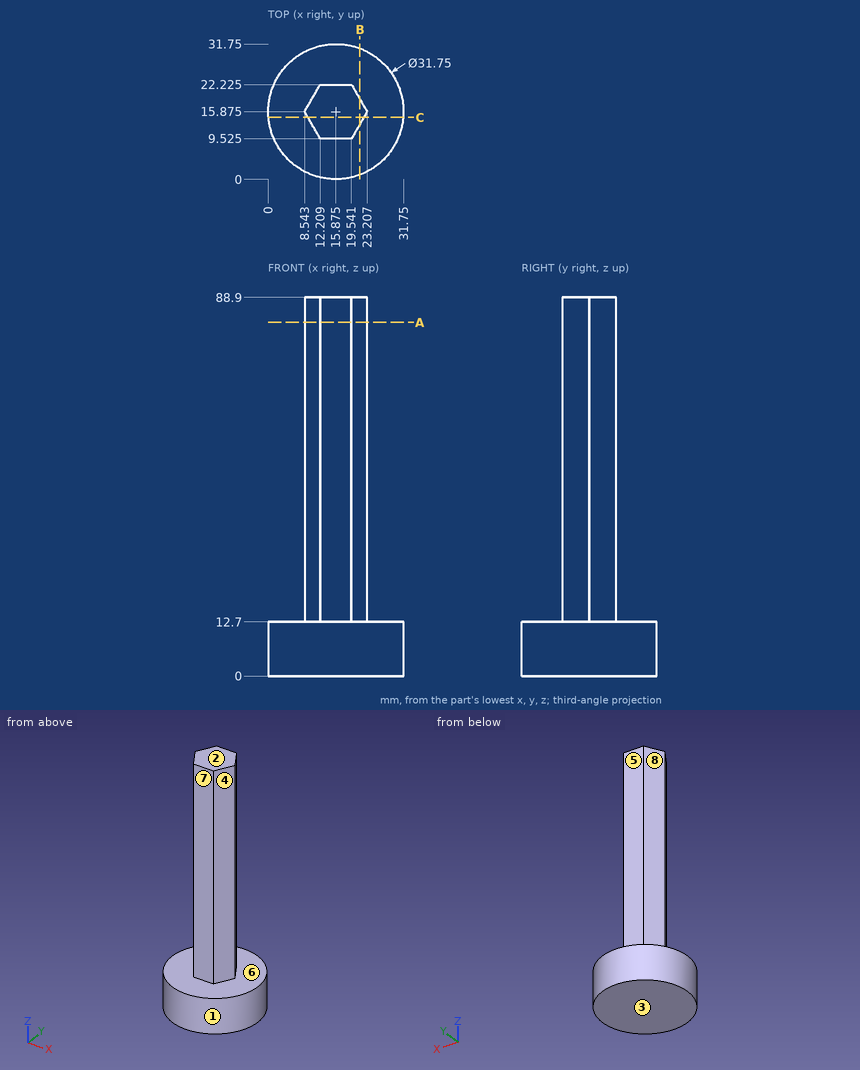
Geometry check sheet. Reference: drawing and pictorial views, mm from the part's lowest x, y, z. A direction names the side the tool comes from. Coordinates: 2 decimals unless noted, no trailing zeros. Order: outer loops, then holes, each group sorted by start corner. A loop starts at its lowest first (then second) coordinate and runs counter-clockwise, first axis right, second up. Notation, with made-up numbers: (77.5, -0.5) -> (101.5, -0.5) arc R21 cw to (101.5, 11.5) -> close; hole circle Ø2 at (77, 66.5). An arc over 180 degrees is marked (long way). Use CSV: the item, a comma, the result in double quotes. Start each with the question number.
Q1. Section check A-A, the plane z = 83. Record the cut outline in (x, y) (1 decimal), and give its area (3 significant figures).
Q2. Thickness scan on line 1 along Z through (x, y) = (27, 15); line 2 along Y through (x, z) = (13, 61.5) (1 decimal); line 3 along X through (y, z) = (17.5, 31.5). Record the ranges inside material, lowest first.
Q3. Tool access check on the marked faces 4, 5, 6, 7 and 8. Record the directions out of +Z, -Z, +X, -X, +Y, -Y that give a thin tool (end or side, any length) a straight path to the whole face; none if there is none.
Q4. Draft check along Z on the marked faces 1, 2 and 3. Enter one of: +Z half, -Z half, draft (parallel to the pull), parting line (faces both ways), or undercut.
Q5. Section check C-C, the plane y = 14.5. Record the cut outline in (x, z).
Q6. Depth check by flat-ended pin: P1, Ø8, axis at x = 6, y = 5.5, coming from the +Z side; P2, Ø1.5, axis at x = 25.5, z = 15, coming from the -Y side; P3, Ø4, axis at x = 21, z = 37, coming from the -Y side (3 decimals); P4, Ø3, axis at x = 7.5, z = 47, coming from the -Y side. Enter the tip coordinate at first touch or a pass-through.
Q7. Section check B-B, the plane x = 21.5. Record the cut outline in (y, z).
Returned:
1,outline,"(8.5, 15.9) -> (12.2, 9.5) -> (19.5, 9.5) -> (23.2, 15.9) -> (19.5, 22.2) -> (12.2, 22.2) -> close"
1,area,"140 mm^2"
2,line 1,"z = 0 to 12.7"
2,line 2,"y = 9.5 to 22.2"
2,line 3,"x = 9.48 to 22.27"
3,face 4,"+Z, +X, -Y"
3,face 5,"+Z, +X, -X, +Y"
3,face 6,"+Z"
3,face 7,"+Z, +X, -X, -Y"
3,face 8,"+Z, -X, +Y"
4,face 1,"draft"
4,face 2,"+Z half"
4,face 3,"-Z half"
5,outline,"(0.06, 0) -> (31.69, 0) -> (31.69, 12.7) -> (22.41, 12.7) -> (22.41, 88.9) -> (9.34, 88.9) -> (9.34, 12.7) -> (0.06, 12.7) -> close"
6,P1,"stops at z = 12.7"
6,P2,"passes through"
6,P3,"stops at y = 9.525"
6,P4,"stops at y = 15.08"
7,outline,"(1.03, 0) -> (30.72, 0) -> (30.72, 12.7) -> (18.83, 12.7) -> (18.83, 88.9) -> (12.92, 88.9) -> (12.92, 12.7) -> (1.03, 12.7) -> close"
